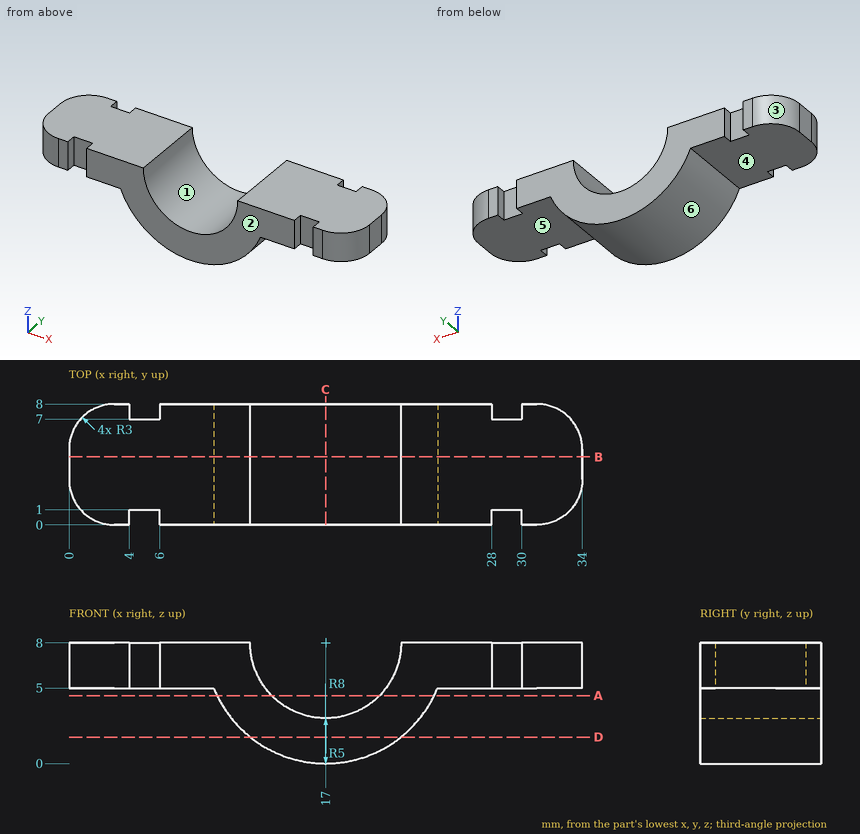
Answer from the drawing. Dimensions are ordinates in mm from the lowest x, y and z of the part. A direction names the side the tool comes from. Round coordinates to 2 decimals unless told otherwise and drop trailing zeros. Loops run counter-clockwise (first coordinate to the right, second up) from the corner with the lowest first, then second, coordinate; pieces in that order, holes last.
(1) Find the intervals of material crossed by L1, parallel to X at y = 4.25, z = 7.75; L2, parallel to Z at x = 9.5, y = 0.75; L3, parallel to X at y = 5.25, z = 6.5, in increasing order.
Computed values:
L1: x = 0 to 12.01, 21.99 to 34
L2: z = 5 to 8
L3: x = 0.01 to 12.23, 21.77 to 33.99
(2) The part is cut by section D-D, the plane z = 1.75. Give the vertices of the cut face in (x, y).
Computed values:
outline: (12.01, 0) - (21.99, 0) - (21.99, 8) - (12.01, 8) - close
(3) The part is cut by section C-C, the plane x = 17. Give the vertices of the cut face in (y, z).
Computed values:
outline: (0, 0) - (8, 0) - (8, 3) - (0, 3) - close
(4) The mould has two halves that part along X. Classify the marked faces 1, 2 and 3: pulls with the +X half, pulls with the -X half, needs draft (parallel to the pull), parting line crosses it, or undercut.
Computed values:
face 1: undercut
face 2: needs draft
face 3: pulls with the -X half
(5) Each of these flat-tipped pins is pushed along its axis until it touches: P1, Ø0.8, axis at y = 0.5, z = 6, coming from the -X side; P2, Ø1.5, axis at y = 7, z = 6, coming from the +X side; P3, Ø3, axis at x = 14.5, z = 5, coming from the +Y side; P4, Ø1, axis at x = 29, z = 7, coming from the -Y side. Where does it stop, or does it pass through?
Computed values:
P1: stops at x = 0.86
P2: stops at x = 33.73
P3: stops at y = 8
P4: stops at y = 1
(6) The part is cut by section B-B, the plane y = 4.5. Give the vertices of the cut face in (x, z).
Computed values:
outline: (0, 5) - (9.58, 5) arc R8 ccw to (24.42, 5) - (34, 5) - (34, 8) - (22, 8) arc R5 cw to (12, 8) - (0, 8) - close
(7) The part is cut by section A-A, the plane z = 4.5. Give the vertices of the cut face in (x, y), and give its area (3 significant figures).
Computed values:
outline: (9.81, 0) - (13.43, 0) - (13.43, 8) - (9.81, 8) - close; (20.57, 0) - (24.19, 0) - (24.19, 8) - (20.57, 8) - close
area: 58.0 mm2
(8) For the marked faces 4, 5 and 6, determine the directions among +Z, -Z, +X, -X, +Y, -Y from which every point of the face is accessible in a straight line to the end or side of a thin tool.
Computed values:
face 4: -Z, -X, +Y, -Y
face 5: -Z, +X, +Y, -Y
face 6: -Z, +Y, -Y
